Source: CAD feature listing. Evaluate the final solid. Frame: model axes, mm. A direction names the side the tool comes from. Give positions to 0.01 mm unless a question says otherwise; leave off trailing zeros. Order: outer loops, then holes, each group sorted by start corner. A loop starts at its lowest first (then second) coordinate and runs counter-clockwise, first axis right, second up.
from build123d import *

# Parameters (mm, degrees)
F0_W     = 50.8
F0_H     = 50.8
F1_DEPTH = 50.8
F3_DEPTH = 25.4
F4_W     = 25.4
F4_H     = 25.4
F5_DEPTH = 25.4
F6_R     = 2.54


with BuildPart() as f1:
    # F0 (on Front) → F1 (new body)
    with BuildSketch(Plane.XZ):
        with Locations((25.4, 25.4)):
            Rectangle(F0_W, F0_H)
    extrude(amount=F1_DEPTH)

    # F2 (on face) → F3 (cut)
    with BuildSketch(Plane.XY.offset(50.8)):
        Polygon((50.8, 0), (25.4, 0), (25.4, -25.4), (0, -25.4), (0, -50.8), (50.8, -50.8), align=None)
    extrude(amount=-F3_DEPTH, mode=Mode.SUBTRACT)

    # F4 (on face) → F5 (cut)
    with BuildSketch(Plane.XY.offset(25.4)):
        with Locations((38.1, -38.1)):
            Rectangle(F4_W, F4_H)
    extrude(amount=-F5_DEPTH, mode=Mode.SUBTRACT)

    # F6
    f6_edges = [f1.edges().sort_by_distance(p)[0] for p in [
        (50.8, -12.7, 25.4),
        (0, -38.1, 25.4),
        (25.4, -12.7, 50.8),
        (12.7, -25.4, 50.8),
        (0, -12.7, 50.8),
        (12.7, 0, 50.8),
        (38.1, 0, 25.4),
        (25.4, 0, 38.1),
        (12.7, -50.8, 25.4),
        (12.7, -50.8, 0),
        (38.1, -25.4, 0),
        (50.8, -25.4, 12.7),
        (25.4, -50.8, 12.7),
        (0, -50.8, 12.7),
        (25.4, 0, 0),
        (50.8, -12.7, 0),
        (0, 0, 25.4),
        (0, -25.4, 0),
        (50.8, 0, 12.7),
        (0, -25.4, 38.1),
    ]]
    fillet(f6_edges, radius=F6_R)


solid = f1.part
(1) Pin query (flat end, axial travel): pin 1 Ø25 at (x, z) = (16.5, 38) entering from -Y; pin 2 Ø2 at (y, z) = (-8.5, 43) entering from +X; pin 3 Ø7 at (x, y) = (41, -8.5) entering from +Z. Return the tip coordinate at first contact, or that it passes through.
(2) Section A-A, the plane z = 42. Return loops of the section in (x, y), plus the area to 3 significant figures.
(3) Section B-B, the plane x = 35.5. Return loops of the section in (y, z), plus the area to 3 significant figures.
(4) Draft query along X for faces 1 (the cylindrical face through (14.13, -50.036, 24.676)), 2 (the cylindrical face through (0.724, -25.72, 0.764)), 3 (the cylindrical face through (24.636, -50.076, 12.522)). Return one class per face: +X half, -X half, draft (parallel to the pull), parting line (faces both ways), or undercut.
(5) Access query for faces 4 (the flat face through (14, -37, 25.4)), 5 (the flat face through (37, -25.4, 14)), 6 (the cylindrical face through (50.036, -12.842, 0.724)). Directions: +Z, -Z, +X, -X, +Y, -Y. A direction counts if a zero-diameter tool reaches every point of the face in a straight line with its end or side. Return the directions, or none.
(6) Section D-D, the plane x = 16.5. Return loops of the section in (y, z).
(7) Section C-C, the plane y = -26.5. Return loops of the section in (x, z).
(8) Line query: line 1 along X through (y, z) = (-26, 11.5); line 2 along Y through (x, z) = (13.5, 38). Output: solid intervals per line, ascending.
Checks:
1. pin 1: stops at y = -25.4
1. pin 2: stops at x = 25.4
1. pin 3: stops at z = 25.4
2. outline: (0, -22.86) arc R2.54 ccw to (2.54, -25.4) - (25.4, -25.4) - (25.4, -2.54) arc R2.54 ccw to (22.86, 0) - (2.54, 0) arc R2.54 ccw to (0, -2.54) - close
2. area: 641 mm2
3. outline: (-25.4, 2.54) arc R2.54 ccw to (-22.86, 0) - (-2.54, 0) arc R2.54 ccw to (0, 2.54) - (0, 22.86) arc R2.54 ccw to (-2.54, 25.4) - (-25.4, 25.4) - close
3. area: 641 mm2
4. face 1: draft
4. face 2: -X half
4. face 3: +X half
5. face 4: +Z, +X, -X, -Y
5. face 5: +Z, -Z, +X, -Y
5. face 6: -Z, +X, +Y, -Y
6. outline: (-50.8, 2.54) arc R2.54 ccw to (-48.26, 0) - (-2.54, 0) arc R2.54 ccw to (0, 2.54) - (0, 48.26) arc R2.54 ccw to (-2.54, 50.8) - (-22.86, 50.8) arc R2.54 ccw to (-25.4, 48.26) - (-25.4, 25.4) - (-48.26, 25.4) arc R2.54 ccw to (-50.8, 22.86) - close
7. outline: (0, 2.54) arc R2.54 ccw to (2.54, 0) - (25.4, 0) - (25.4, 25.4) - (2.54, 25.4) arc R2.54 ccw to (0, 22.86) - close
8. line 1: x = 0 to 25.4
8. line 2: y = -25.4 to 0
